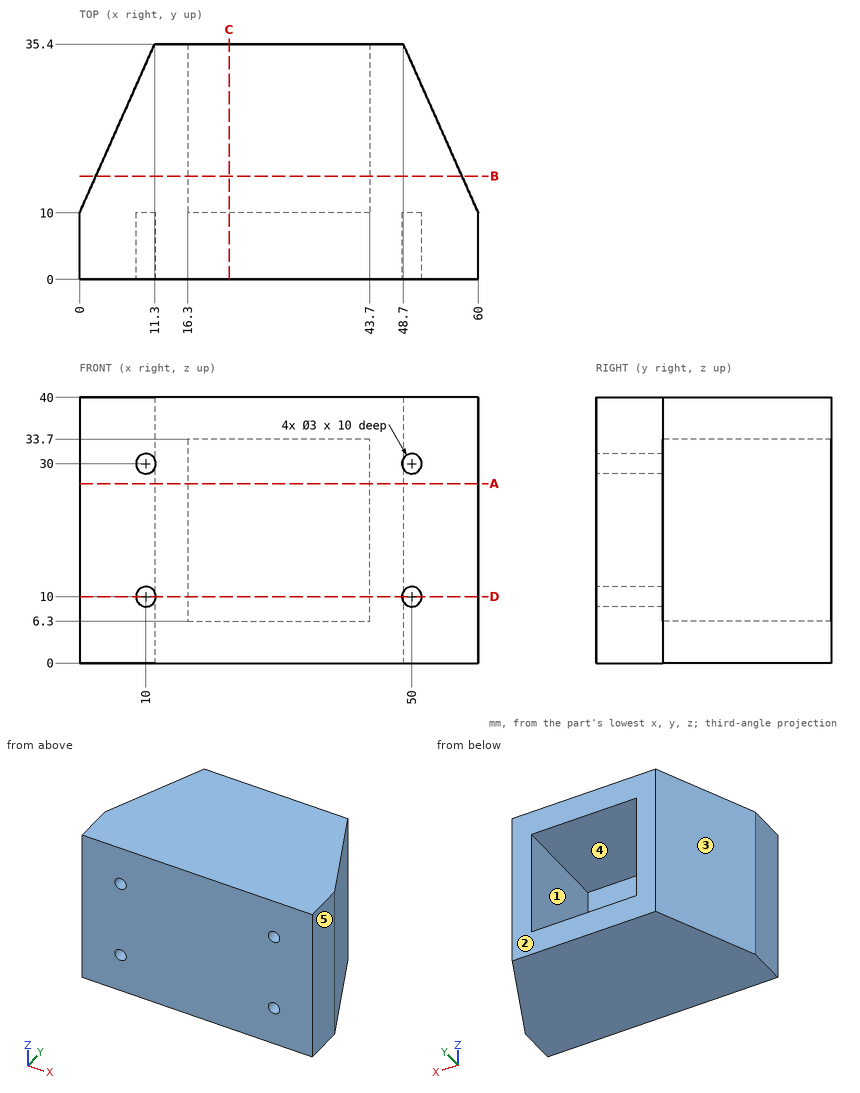
Print and shaded views of the part. All mm, measured from the part's lowest x, y and z. A direction names the side the tool comes from. Round coordinates to 2 decimals unless told otherwise and drop trailing zeros. Write each loop counter-clockwise with the first axis right and the second up, starting at its lowest first coordinate (ties: lowest second). Pieces come first, ordered by that corner, then holes. Notation, with made-up numbers: (8, -28.5) -> (16, -28.5) arc R5 ccw to (16, -19.5) -> close; hole circle Ø8 at (83, 37). An arc over 180 degrees is marked (long way). Answer in a Markdown table with one row per item. Add a question column.
Item 1: Drop flat-ended pins along their axis: pin 1 Ø0.9 at (x, z) = (10, 29.5) entering from -Y; pin 2 Ø3 at (y, z) = (27.5, 4) entering from +X; pin 3 Ø3.5 at (x, z) = (50, 30) entering from +Y; pin 4 Ø12.5 at (y, z) = (21, 25.5) entering from +X. Give the stop position or say it passes through.
Item 2: Which spindle directions (+Z, -Z, +X, -X, +Y, -Y) get a long thin tool onto all of the face, cutting with end or side? Do the marked faces 4 and 5. Say none if no direction does.
Item 3: Saw through at C-C, the plane x = 22.5. Write the cut outline in (y, z).
Item 4: Saw through at B-B, the plane y = 15.5. Write the cut outline in (x, z).
Item 5: Mould opens along X. For the marked faces 1, 2 and 3 say: pulls with the +X half, pulls with the -X half, needs draft (parallel to the pull), parting line crosses it, or undercut.
Item 6: Saw through at D-D, the plane z = 10. Write the cut outline in (x, y).
Item 7: Saw through at A-A, the plane z = 27. Write the cut outline in (x, y), then the cut area to 3 significant figures.
Item 8: Drill centre lines: line 1 (Z direction, x = 10, y = 2.5); line 2 (Z direction, x = 28, y = 24.5); line 3 (X direction, y = 15, z = 25). Where is each one in solid material? Low to high. Write a range as from..to.
Findings below:
| question | item | result |
|---|---|---|
| 1 | pin 1 | stops at y = 10 |
| 1 | pin 2 | stops at x = 52.88 |
| 1 | pin 3 | stops at y = 35.4 |
| 1 | pin 4 | stops at x = 57.89 |
| 2 | face 4 | +Y |
| 2 | face 5 | +Z, -Z, +X, +Y, -Y |
| 3 | outline | (0, 0) -> (35.4, 0) -> (35.4, 6.3) -> (10, 6.3) -> (10, 33.7) -> (35.4, 33.7) -> (35.4, 40) -> (0, 40) -> close |
| 4 | outline | (2.45, 0) -> (57.55, 0) -> (57.55, 40) -> (2.45, 40) -> close; hole (16.3, 6.3) -> (43.7, 6.3) -> (43.7, 33.7) -> (16.3, 33.7) -> close |
| 5 | face 1 | undercut |
| 5 | face 2 | needs draft |
| 5 | face 3 | pulls with the -X half |
| 6 | outline | (0, 0) -> (8.5, 0) -> (8.5, 10) -> (11.5, 10) -> (11.5, 0) -> (48.5, 0) -> (48.5, 10) -> (51.5, 10) -> (51.5, 0) -> (60, 0) -> (60, 10) -> (48.7, 35.4) -> (43.7, 35.4) -> (43.7, 10) -> (16.3, 10) -> (16.3, 35.4) -> (11.3, 35.4) -> (0, 10) -> close |
| 7 | outline | (0, 0) -> (60, 0) -> (60, 10) -> (48.7, 35.4) -> (43.7, 35.4) -> (43.7, 10) -> (16.3, 10) -> (16.3, 35.4) -> (11.3, 35.4) -> (0, 10) -> close |
| 7 | area | 1,140 mm^2 |
| 8 | line 1 | z = 0..8.5, 11.5..28.5, 31.5..40 |
| 8 | line 2 | z = 0..6.3, 33.7..40 |
| 8 | line 3 | x = 2.22..16.3, 43.7..57.78 |
